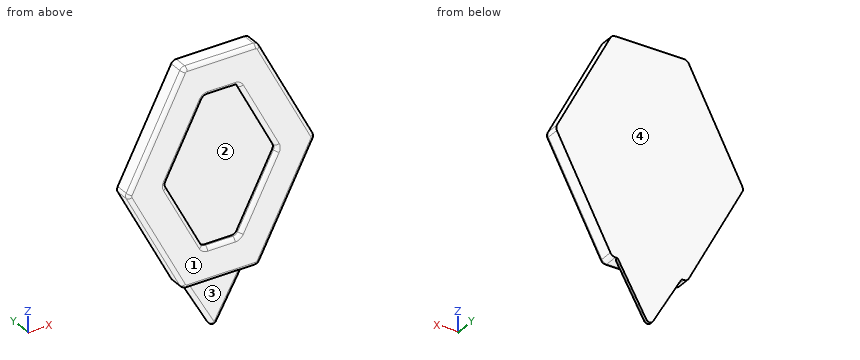
```python
from build123d import *

# Parameters (mm, degrees)
F1_DEPTH = 3
F3_DEPTH = 3
F5_DEPTH = 3
F6_R     = 3
F7_R     = 2


with BuildPart() as f1:
    # F0 (on Front) → F1 (new body)
    with BuildSketch(Plane.XZ):
        Polygon((20, 51.98047), (0, 51.98047), (-20, 51.98047), (-50, -5.682343), (-20, -63.01953), (-17, -63.01953), (0, -63.01953), (17, -63.01953), (20, -63.01953), (50, -5.682343), align=None)
        Polygon((0, -93.01953), (17, -63.01953), (0, -63.01953), (-17, -63.01953), align=None)
    extrude(amount=F1_DEPTH)

    # F2 (on face) → F3 (join)
    with BuildSketch(Plane.XZ.offset(3)):
        Polygon((20, 51.98047), (-20, 51.98047), (-50, -5.682343), (-20, -63.01953), (20, -63.01953), (50, -5.682343), align=None)
    extrude(amount=F3_DEPTH)

    # F4 (on face) → F5 (join)
    with BuildSketch(Plane.XZ.offset(6)):
        Polygon((20, 51.98047), (-20, 51.98047), (-50, -5.682343), (-20, -63.01953), (20, -63.01953), (50, -5.682343), align=None)
        Polygon((-9.102997, -45.01953), (-29.697361, -5.658767), (-9.074414, 33.98047), (9.074414, 33.98047), (29.697361, -5.658767), (9.102997, -45.01953), align=None, mode=Mode.SUBTRACT)
    extrude(amount=F5_DEPTH)

    # F6
    f6_edges = [f1.edges().sort_by_distance(p)[0] for p in [
        (-20, -4.5, 51.98047),
        (20, -4.5, 51.98047),
        (-50, -4.5, -5.682343),
        (-20, -4.5, -63.01953),
        (20, -4.5, -63.01953),
        (50, -4.5, -5.682343),
        (9.074414, -7.5, 33.98047),
        (29.697361, -7.5, -5.658767),
        (-9.074414, -7.5, 33.98047),
        (-29.697361, -7.5, -5.658767),
        (-9.102997, -7.5, -45.01953),
        (9.102997, -7.5, -45.01953),
    ]]
    fillet(f6_edges, radius=F6_R)

    # F7
    f7_edges = [f1.edges().sort_by_distance(p)[0] for p in [
        (-35.059009, -9, 23.035643),
        (-19.444896, -9, 14.047431),
        (8.5, -3, -78.01953),
        (-8.5, -3, -78.01953),
        (0, -1.5, -93.01953),
    ]]
    fillet(f7_edges, radius=F7_R)


solid = f1.part
```
Verification items for the finished model (mm, model axes). Face numbers are marked on the shaded views. A direction names the side the tool comes from. Coordinates: 2 decimals unless noted, no trailing zeros. Answer as a JSON object with one key per item and string values.
(1) Scan lines: line 1 along Z through (x, y) = (13, -7.25); line 2 along Z through (x, y) = (3, -7.25); line 3 along X through (y, z) = (-8, -41.5). Record each from-to range of solid material in increasing order.
Response:
{"line 1": "z = -63 to -37.61, 26.47 to 51.96", "line 2": "z = -63 to -45.04, 34 to 51.96", "line 3": "x = -30.96 to -11.25, 11.25 to 30.96"}
(2) Access from +Z, -Z, +X, -X, +Y, -Y to the whole of each face (thin tool, end or side, straight path). Record for the marked faces 3 and 4.
Response:
{"face 3": "-Z, +X, -X, -Y", "face 4": "+Z, -Z, +X, -X, +Y"}
(3) Go/stop test with flat-tipped pins: pin 1 Ø4 at (y, z) = (-4, -32.5) entering from -X; pin 2 Ø8 at (x, z) = (-2.5, -82) entering from -Y; pin 3 Ø0.8 at (x, y) = (0, -6.5) entering from -Z. Record where each tip stops, or that it passes through.
Response:
{"pin 1": "stops at x = -37.01", "pin 2": "stops at y = -3", "pin 3": "stops at z = -63.02"}
(4) Mould release check, pull along Z, two halves, no side actions. Record for the marked faces 1 and 2: pulls with the +Z half, pulls with the -Z half, needs draft (parallel to the pull), parting line crosses it, or undercut.
Response:
{"face 1": "needs draft", "face 2": "undercut"}
